Input: part model. Units: mm. Frame: model coordinates. A direction names the side the tool comes from. Coordinates: 2 decimals unless noted, no trailing zeros. Order: outer loops, then holes, each group sorted by start corner. A loop starts at its lowest first (then second) coordinate and runs counter-clockwise, first axis right, second up.
from build123d import *

# Parameters (mm, degrees)
SKETCH_1_W          = 50
SKETCH_1_H          = 105
EXTRUDE_1_DEPTH     = 4
SKETCH_2_R          = 1.15
CUT_EXTRUDE_1_DEPTH = 5
CUT_EXTRUDE_2_DEPTH = 1.5
SKETCH_4_R          = 2.25
CUT_EXTRUDE_3_DEPTH = 1.5
SKETCH_5_R          = 1.15
CUT_EXTRUDE_4_DEPTH = 3.5
SKETCH_6_W          = 5
SKETCH_6_H          = 10
EXTRUDE_2_DEPTH     = 4
SKETCH_7_R          = 1.75
CUT_EXTRUDE_5_DEPTH = 5
SKETCH_8_R          = 13
SKETCH_8_R_2        = 9
CUT_EXTRUDE_6_DEPTH = 5
FILLET_1_R          = 1.5


with BuildPart() as part:
    # 草图1 → 凸台-拉伸1 (new body)
    with BuildSketch(Plane(origin=(0, 0, 0), x_dir=(1, 0, 0), z_dir=(0, 1, 0))):
        with Locations((76.431630633, 94.447783849)):
            Rectangle(SKETCH_1_W, SKETCH_1_H)
    extrude(amount=EXTRUDE_1_DEPTH)

    # 草图2 → 切除-拉伸1 (cut)
    with BuildSketch(Plane(origin=(0, 4, 0), x_dir=(1, 0, 0), z_dir=(0, 1, 0))):
        with Locations((72.181630633, 88.447783849)):
            Circle(SKETCH_2_R)
        with Locations((72.181630633, 47.447783849)):
            Circle(SKETCH_2_R)
        with Locations((80.681630633, 47.447783849)):
            Circle(SKETCH_2_R)
        with Locations((80.681630633, 88.447783849)):
            Circle(SKETCH_2_R)
    extrude(amount=-CUT_EXTRUDE_1_DEPTH, mode=Mode.SUBTRACT)

    # 草图3 → 切除-拉伸2 (cut)
    with BuildSketch(Plane(origin=(0, 4, 0), x_dir=(1, 0, 0), z_dir=(0, 1, 0))):
        with BuildLine():
            Line((72.181630633, 91.247783849), (80.681630633, 91.247783849))
            ThreePointArc((80.681630633, 91.247783849), (83.481630633, 88.447783849), (80.681630633, 85.647783849))
            Line((80.681630633, 85.647783849), (72.181630633, 85.647783849))
            ThreePointArc((72.181630633, 85.647783849), (69.381630633, 88.447783849), (72.181630633, 91.247783849))
        make_face()
        with BuildLine():
            Line((80.681630633, 44.647783849), (72.181630633, 44.647783849))
            ThreePointArc((72.181630633, 44.647783849), (69.381630633, 47.447783849), (72.181630633, 50.247783849))
            Line((72.181630633, 50.247783849), (80.681630633, 50.247783849))
            ThreePointArc((80.681630633, 50.247783849), (83.481630633, 47.447783849), (80.681630633, 44.647783849))
        make_face()
    extrude(amount=-CUT_EXTRUDE_2_DEPTH, mode=Mode.SUBTRACT)

    # 草图4 → 切除-拉伸3 (cut)
    with BuildSketch(Plane(origin=(0, 4, 0), x_dir=(1, 0, 0), z_dir=(0, 1, 0))):
        with Locations((86.431630633, 130.947783849)):
            Circle(SKETCH_4_R)
        with Locations((86.431630633, 110.947783849)):
            Circle(SKETCH_4_R)
        with Locations((66.431630633, 110.947783849)):
            Circle(SKETCH_4_R)
        with Locations((66.431630633, 130.947783849)):
            Circle(SKETCH_4_R)
    extrude(amount=-CUT_EXTRUDE_3_DEPTH, mode=Mode.SUBTRACT)

    # 草图5 → 切除-拉伸4 (cut, through all)
    with BuildSketch(Plane(origin=(0, 2.5, 0), x_dir=(1, 0, 0), z_dir=(0, 1, 0))):
        with Locations((66.431630633, 130.947783849)):
            Circle(SKETCH_5_R)
        with Locations((86.431630633, 130.947783849)):
            Circle(SKETCH_5_R)
        with Locations((66.431630633, 110.947783849)):
            Circle(SKETCH_5_R)
        with Locations((86.431630633, 110.947783849)):
            Circle(SKETCH_5_R)
    extrude(amount=-CUT_EXTRUDE_4_DEPTH, mode=Mode.SUBTRACT)

    # 草图6 → 凸台-拉伸2 (add)
    with BuildSketch(Plane(origin=(0, 4, 0), x_dir=(1, 0, 0), z_dir=(0, 1, 0))):
        with Locations((103.931630633, 46.947783849)):
            Rectangle(SKETCH_6_W, SKETCH_6_H)
        with Locations((48.931630633, 46.947783849)):
            Rectangle(SKETCH_6_W, SKETCH_6_H)
        with Locations((48.931630633, 141.947783849)):
            Rectangle(SKETCH_6_W, SKETCH_6_H)
        with Locations((103.931630633, 141.947783849)):
            Rectangle(SKETCH_6_W, SKETCH_6_H)
    extrude(amount=-EXTRUDE_2_DEPTH)

    # 草图7 → 切除-拉伸5 (cut, through all)
    with BuildSketch(Plane(origin=(0, 4, 0), x_dir=(1, 0, 0), z_dir=(0, 1, 0))):
        with Locations((102.931630633, 46.947783849)):
            Circle(SKETCH_7_R)
        with Locations((49.931630633, 46.947783849)):
            Circle(SKETCH_7_R)
        with Locations((49.931630633, 141.947783849)):
            Circle(SKETCH_7_R)
        with Locations((102.931630633, 141.947783849)):
            Circle(SKETCH_7_R)
    extrude(amount=-CUT_EXTRUDE_5_DEPTH, mode=Mode.SUBTRACT)

    # 草图8 → 切除-拉伸6 (cut, through all)
    with BuildSketch(Plane(origin=(0, 4, 0), x_dir=(1, 0, 0), z_dir=(0, 1, 0))):
        with Locations((76.431630633, 67.947783849)):
            Circle(SKETCH_8_R)
        with Locations((76.431630633, 120.947783849)):
            Circle(SKETCH_8_R_2)
    extrude(amount=-CUT_EXTRUDE_6_DEPTH, mode=Mode.SUBTRACT)

    # 圆角1
    fillet_1_edges = [part.edges().sort_by_distance(p)[0] for p in [
        (106.431630633, 2, -146.947783849),
        (106.431630633, 2, -136.947783849),
        (101.431630633, 2, -136.947783849),
        (51.431630633, 2, -136.947783849),
        (46.431630633, 2, -136.947783849),
        (46.431630633, 2, -146.947783849),
        (51.431630633, 2, -51.947783849),
        (46.431630633, 2, -41.947783849),
        (46.431630633, 2, -51.947783849),
        (106.431630633, 2, -41.947783849),
        (101.431630633, 2, -51.947783849),
        (106.431630633, 2, -51.947783849),
    ]]
    fillet(fillet_1_edges, radius=FILLET_1_R)


solid = part.part
Item 1: Cut plane C-C on z = -105. Return loops of the section in (x, y), then the cut area to 3 significant figures.
Response values:
outline: (51.43, 0) - (101.43, 0) - (101.43, 4) - (51.43, 4) - close
area: 200 mm2
Item 2: Cut plane A-A on z = -58. Return loops of the section in (x, y).
Response values:
outline: (51.43, 0) - (68.06, 0) - (68.06, 4) - (51.43, 4) - close; (84.8, 0) - (101.43, 0) - (101.43, 4) - (84.8, 4) - close
Item 3: Cut plane B-B on y = 1.35. Count the separate pieces of the cut face and the enclosed holes in it, then the cut area to 3 significant figures.
Response values:
separate pieces: 1
enclosed holes: 14
area: 4,590 mm2
Item 4: Draft query along X for faces 4 (the face through (66.282, 1.268, -132.088)), 5 (the face through (51.432, 2, -94)), 6 (the face through (104, 2, -136.948)). Return one class per face: pulls with the +X half, pulls with the -X half, needs draft (parallel to the pull), parting line crosses it, or undercut.
Response values:
face 4: undercut
face 5: pulls with the -X half
face 6: needs draft
Item 5: Access query for faces 1 (the face through (69.382, 3.26, -47.386)), 2 (the face through (49, 2, -136.948)), 3 (the face through (79.834, 1.268, -89.225)). Directions: +Z, -Z, +X, -X, +Y, -Y. A direction counts if a zero-diameter tool reaches every point of the face in a straight line with its end or side. Return the directions, or none.
Response values:
face 1: +Y
face 2: -X, +Y, -Y
face 3: +Y, -Y
Item 6: Pin query (flat end, axial travel): pin 1 Ø2 at (x, z) = (86, -130.5) entering from +Y; pin 2 Ø2 at (x, z) = (72.18, -88.45) entering from -Y; pin 3 Ø1 at (y, z) = (0.5, -108.5) entering from -X. Return the tip coordinate at first contact, or that it passes through.
Response values:
pin 1: stops at y = 2.5
pin 2: passes through
pin 3: stops at x = 51.43
Item 7: Ray query, probe 1 along Z at (x, y) = (76.5, 1.25); probe 2 along Z at (x, y) = (74, 3.8); probe 3 along Z at (x, y) = (104.5, 2.7). Return the intervals inside material, ascending.
Response values:
probe 1: z = -146.95 to -129.95, -111.95 to -80.95, -54.95 to -41.95
probe 2: z = -146.95 to -129.61, -112.28 to -91.25, -85.65 to -80.72, -55.18 to -50.25, -44.65 to -41.95
probe 3: z = -146.95 to -142.72, -141.17 to -136.95, -51.95 to -47.72, -46.17 to -41.95
